For this review, use the dimensioned drawing (mm, ordinates from the lowest corner) and the shaded views. A direction names the side the tool comes from. Give positions to 0.01 mm unless a question says otherwise; leave off trailing zeros. Write each loop counter-clockwise with the first axis right and the second up, starting at its lowest first coordinate (ties: lowest second). Pieces come first, ordered by that corner, then holes. Notation, with made-up numbers: M 69.25,87.25 L 115.25,87.25 A23 ccw 115.25,120.25 Z; hole C 61,67 d10. An arc over 180 degrees is marked long. One line per item, written item: value. Start each with the question number.
Item 1: Consider section C-C, the plane y = 225. Write out the cut boundary in (x, z), and give its area (3 significant figures).
Item 2: Clearance check with flat-ended pins moving along their axes: pin 1 Ø12 at (x, y) = (204.5, 172) entering from -Z; pin 2 Ø20 at (y, z) = (20, 30) entering from +X; pin 3 Ø3 at (x, y) = (109.5, 234.5) entering from +Z. State where each tip first meets the part, or that it passes through.
Item 3: Consider section B-B, the plane z = 80. Write out the cut boundary in (x, y), and give its area (3 significant figures).
Item 4: Tool access review of the marked faces 1 and 2: name each direction out of +Z, -Z, +X, -X, +Y, -Y from which nothing blocks a thin tool from reaching the whole face with its end or side.
Item 5: To check wall thickness, follow probe 1 along Z at (x, y) = (7.5, 300); probe 2 along Z at (x, y) = (2.75, 20); probe 3 along Z at (x, y) = (50, 85). State the ranges of each line that lie inside material, in increasing order.
Item 6: Consider section A-A, the plane y = 300. Write out the cut boundary in (x, z), and give its area (3 significant figures).
Item 7: Consider section D-D, the plane x = 128. Write out the cut boundary in (y, z), and give its area (3 significant figures).
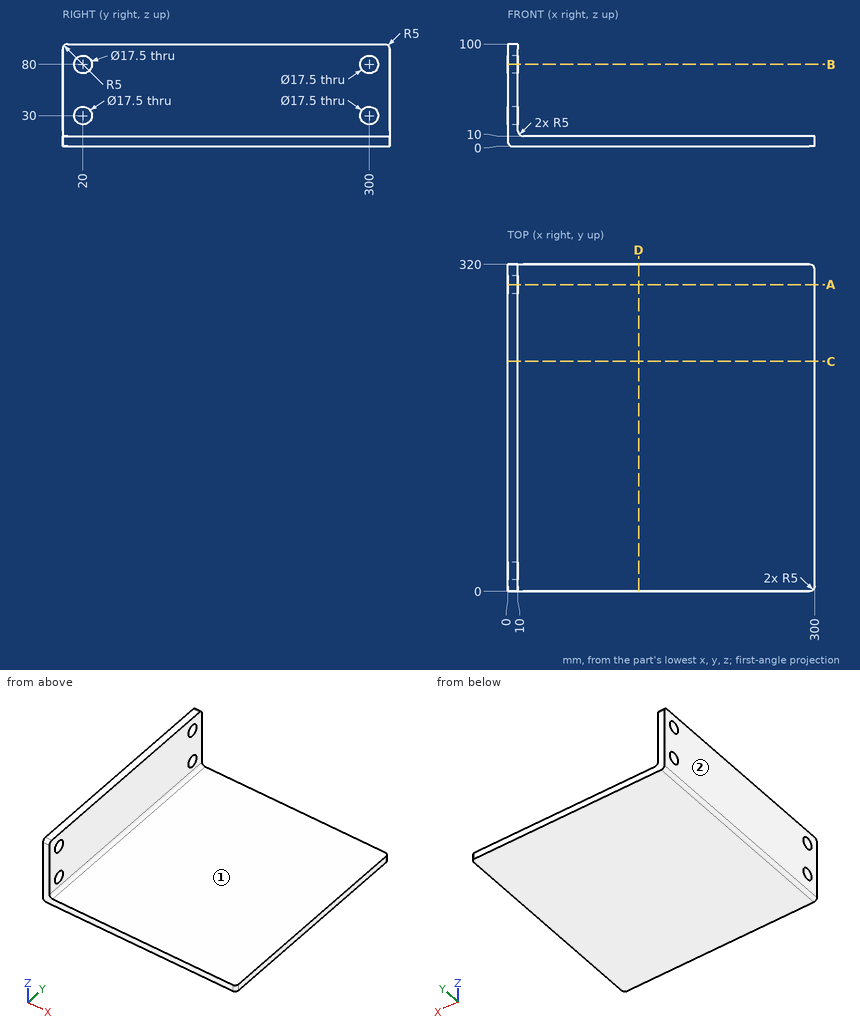
Model answer:
1. outline: M 0,5 A5 ccw 5,0 L 300,0 L 300,10 L 15,10 A5 cw 10,15 L 10,100 L 0,100 Z
1. area: 3,900 mm2
2. pin 1: stops at z = 0
2. pin 2: stops at x = 10
2. pin 3: stops at z = 10
3. outline: M 0,0 L 10,0 L 10,11.25 L 0,11.25 Z; M 0,28.75 L 10,28.75 L 10,291.25 L 0,291.25 Z; M 0,308.75 L 10,308.75 L 10,320 L 0,320 Z
3. area: 2,850 mm2
4. face 1: +Z, +X, +Y, -Y
4. face 2: +Z, -Z, -X, +Y, -Y
5. probe 1: z = 0 to 21.25, 38.75 to 71.25, 88.75 to 100
5. probe 2: z = 0.53 to 21.25, 38.75 to 71.25, 88.75 to 100
5. probe 3: z = 0 to 10
6. outline: M 0,5 A5 ccw 5,0 L 300,0 L 300,10 L 15,10 A5 cw 10,15 L 10,21.25 L 0,21.25 Z; M 0,38.75 L 10,38.75 L 10,71.25 L 0,71.25 Z; M 0,88.75 L 10,88.75 L 10,100 L 0,100 Z
6. area: 3,550 mm2
7. outline: M 0,0 L 320,0 L 320,10 L 0,10 Z
7. area: 3,200 mm2
